```python
from build123d import *

# Parameters (mm, degrees)
F1_DEPTH = 63.5
F0_W     = 25.4
F0_H     = 19.05
F2_DEPTH = 25.4
F3_DEPTH = 7.9375
F5_R     = 5.08
F7_D     = 12.7
F8_SIZE  = 2.54


with BuildPart() as f1:
    # F0 (on Front) → F1 (new body, symmetric)
    with BuildSketch(Plane.XZ):
        Polygon((22.225, 9.525), (-41.275, 9.525), (-41.275, -9.525), (41.275, -9.525), (41.275, 9.525), align=None)
    extrude(amount=F1_DEPTH, both=True)

    # F0 (on Front) → F2 (join, symmetric)
    with BuildSketch(Plane.XZ):
        with BuildLine():
            Line((22.225, 27.0002), (22.225, 9.525))
            Line((22.225, 9.525), (41.275, 9.525))
            Line((41.275, 9.525), (41.275, 27.0002))
            ThreePointArc((41.275, 27.0002), (45.9246798487, 38.2255201513), (57.15, 42.8752))
            Line((57.15, 42.8752), (60.325, 42.8752))
            Line((60.325, 42.8752), (60.325, 61.9252))
            Line((60.325, 61.9252), (57.15, 61.9252))
            add(Edge.make_bspline(
                [(53.8854342407, 61.7722898912), (54.9842067368, 61.8365871986), (56.0728453275, 61.8876096574), (57.15, 61.9252)],
                knots=[108.5245810491, 108.5245810491, 108.5245810491, 108.5245810491, 111.5045361635, 111.5045361635, 111.5045361635, 111.5045361635], degree=3))
            ThreePointArc((53.8854342407, 61.7722898912), (31.3258777096, 50.5133948686), (22.225, 27.0002))
        make_face()
        with Locations((73.025, 52.4002)):
            Rectangle(F0_W, F0_H)
    extrude(amount=F2_DEPTH, both=True)

    # F0 (on Front) → F3 (join, symmetric)
    with BuildSketch(Plane.XZ):
        with BuildLine():
            add(Edge.make_bspline(
                [(-41.275, 9.525), (-39.5856284224, 39.4828766469), (13.870125209, 59.4306981306), (53.8854342407, 61.7722898912)],
                knots=[0, 0, 0, 0, 108.5245810491, 108.5245810491, 108.5245810491, 108.5245810491], degree=3))
            Line((-41.275, 9.525), (22.225, 9.525))
            Line((22.225, 9.525), (22.225, 27.0002))
            ThreePointArc((22.225, 27.0002), (31.3258777096, 50.5133948686), (53.8854342407, 61.7722898912))
        make_face()
    extrude(amount=F3_DEPTH, both=True)

    # F0 (on Front) → F4 (revolve)
    with BuildSketch(Plane.XZ):
        Polygon((85.725, 66.675), (85.725, 61.9252), (85.725, 42.8752), (85.725, 38.1), (111.125, 38.1), (111.125, 66.675), align=None)
    revolve(axis=Axis((85.725, 0, 52.3875), (0, 0, 1)))

    # F5
    f5_edges = [f1.edges().sort_by_distance(p)[0] for p in [
        (41.275, -63.5, 0),
        (-41.275, -63.5, 0),
        (41.275, 63.5, 0),
        (-41.275, 63.5, 0),
    ]]
    fillet(f5_edges, radius=F5_R)

    # F7 (through all)
    with Locations(Plane.XY.offset(66.675)):
        with Locations((85.725, 0)):
            Hole(F7_D / 2)

    # F8
    f8_edges = [f1.edges().sort_by_distance(p)[0] for p in [
        (60.325, 0, 66.675),
        (60.325, 0, 38.1),
        (79.375, 0, 66.675),
        (79.375, 0, 38.1),
    ]]
    chamfer(f8_edges, length=F8_SIZE)


solid = f1.part
```
Here's how the part is built. I have some questions about the finished solid (model axes, mm). A direction names the side the tool comes from. Round coordinates to 2 decimals unless told otherwise and drop trailing zeros. Order: outer loops, then holes, each group sorted by start corner. A loop starts at its lowest first (then second) coordinate and runs counter-clockwise, first axis right, second up. Notation, with made-up numbers: M 13.5,58 L 59.5,58 A36 cw 59.5,92 Z; hole C 80,19 d5. An arc over 180 degrees is marked long. Answer as CSV lines item,"result".
Item 1: Imagine slicing it at A-A on y = 43. List the corners of the cut face in (x, z) for me (3 decimals).
From the geometry:
outline,"M -41.275,-9.525 L 41.275,-9.525 L 41.275,9.525 L -41.275,9.525 Z"
Item 2: Which directions (+Z, -Z, +X, -X, +Y, -Y) give clear straight access to the entire face, cutting with the end or side of a thin tool? Please do faces 5 (the flat face through (-4, -7.938, 30)), 6 (the flat face through (60, 2, 42.875)), 7 (the flat face through (86, -10, 38.1)).
From the geometry:
face 5,"+Z, -X, -Y"
face 6,"-Z"
face 7,"-Z, +X, +Y, -Y"
Item 3: For pin 1 (3 mm diameter, centred on x = 28.5, z = 15.5, fed in from +Y); pin 2 (14 mm diameter, centred on y = 20.5, z = 19.5, fed in from -X) (3 decimals); pin 3 (10 mm diameter, centred on x = -12, z = 22.5, fed in from -Y), each with a flat end and sliding along its axis, tell me the tip position at first contact or that it passes through.
From the geometry:
pin 1,"y = 25.4"
pin 2,"x = 22.225"
pin 3,"y = -7.94"
Item 4: Please list where these lines run through material, in increasing order: L1, parallel to X at y = 1.5, z = 41; L2, parallel to Z at x = 29, y = 26 (3 decimals); L3, parallel to Y at x = 16.5, z = 37.5. Write a range as [from, to].
From the geometry:
L1,"[-17.26, 49.67], [60.37, 79.55], [91.9, 111.08]"
L2,"[-9.525, 9.525]"
L3,"[-7.94, 7.94]"
Item 5: We'd pull the mould along X, two halves only. Please class faces 1 (the flat face through (85, -10, 66.675)), 2 (the flat face through (22.225, 17, 18)), 3 (the conical face through (80.743, -22.437, 38.223)), 4 (the conical face through (92.192, 0.285, 64.258)): +X half, -X half, draft (parallel to the pull), parting line (faces both ways), or undercut.
From the geometry:
face 1,"draft"
face 2,"-X half"
face 3,"undercut"
face 4,"undercut"
